The model under review builds one solid part; all positions refer to its coordinate system, in mm. Round coordinates to 2 decimals unless told otherwise and drop trailing zeros. Loops run counter-clockwise (first coordinate to the right, second up) from the corner with the lowest first, then second, coordinate; pieces in that order, holes last. Notation, with made-up numbers: (50.25, 79.5) -> (55.25, 79.5) arc R15 cw to (55.25, 96.5) -> close; hole circle Ø2 at (79, 71). An arc over 180 degrees is marked (long way). Use a Markdown table: item, result. Add a question column.
1) Wall thickness on probe 1 along Z at (x, y) = (23, 8); probe 2 along Y at (x, z) = (-73, -15); probe 3 along Z at (x, y) = (-37, -3.5): over which ranges is each line inside the solid? List them lowest first.
2) Insertion check: pin 1 (3.5 mm diameter, centred on x = 23.32, z = 0.42, fed in from +Y) (3 decimals). The pin has a flat end and moves straight along its axis. Give the tip position at first contact, or say it passes through.
3) Consider section B-B on z = 17.5. Give the boundary of the cut face in (x, y), plus the area to 3 significant figures.
4) Consider section A-A on y = -1.5. Give the boundary of the cut face in (x, z), plus the area to 3 significant figures.
5) Consider section C-C on x = -86.5. Give the boundary of the cut face in (y, z), plus the area to 3 significant figures.
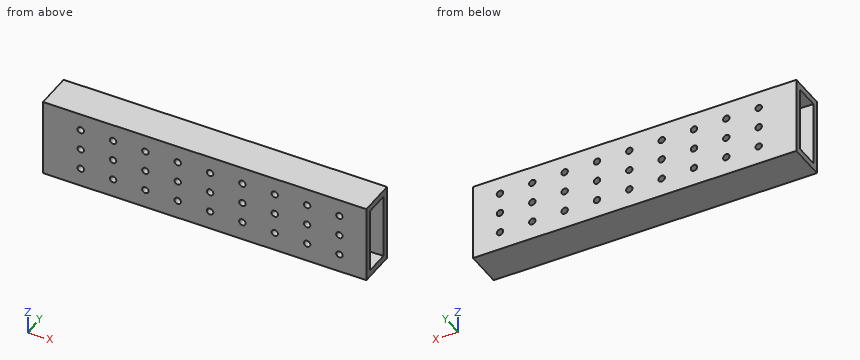
from build123d import *

# Parameters (mm, degrees)
SKETCH1_W           = 48
SKETCH1_H           = 23
SKETCH1_W_2         = 40
SKETCH1_H_2         = 15
EXTRUDE_THIN1_DEPTH = 100
SKETCH2_R           = 2
CUT_EXTRUDE1_DEPTH  = 24


with BuildPart() as part:
    # Sketch1 → Extrude-Thin1 (new body, symmetric)
    with BuildSketch(Plane(origin=(0, 0, 0), x_dir=(0, 0, -1), z_dir=(1, 0, 0))):
        Rectangle(SKETCH1_W, SKETCH1_H)
        Rectangle(SKETCH1_W_2, SKETCH1_H_2, mode=Mode.SUBTRACT)
    extrude(amount=EXTRUDE_THIN1_DEPTH, both=True)

    # Sketch2 → Cut-Extrude1 (cut, through all)
    with BuildSketch(Plane(origin=(0, 11.5, 0), x_dir=(1, 0, 0), z_dir=(0, 1, 0))):
        with Locations((-76.678469137, 12.583133397)):
            Circle(SKETCH2_R)
        with Locations((-56.678469137, 12.583133397)):
            Circle(SKETCH2_R)
        with Locations((-36.678469137, 12.583133397)):
            Circle(SKETCH2_R)
        with Locations((-16.678469137, 12.583133397)):
            Circle(SKETCH2_R)
        with Locations((3.321530863, 12.583133397)):
            Circle(SKETCH2_R)
        with Locations((23.321530863, 12.583133397)):
            Circle(SKETCH2_R)
        with Locations((43.321530863, 12.583133397)):
            Circle(SKETCH2_R)
        with Locations((63.321530863, 12.583133397)):
            Circle(SKETCH2_R)
        with Locations((83.321530863, 12.583133397)):
            Circle(SKETCH2_R)
        with Locations((-56.678469137, -0.416866603)):
            Circle(SKETCH2_R)
        with Locations((-36.678469137, -0.416866603)):
            Circle(SKETCH2_R)
        with Locations((-16.678469137, -0.416866603)):
            Circle(SKETCH2_R)
        with Locations((3.321530863, -0.416866603)):
            Circle(SKETCH2_R)
        with Locations((23.321530863, -0.416866603)):
            Circle(SKETCH2_R)
        with Locations((43.321530863, -0.416866603)):
            Circle(SKETCH2_R)
        with Locations((63.321530863, -0.416866603)):
            Circle(SKETCH2_R)
        with Locations((83.321530863, -0.416866603)):
            Circle(SKETCH2_R)
        with Locations((-56.678469137, -13.416866603)):
            Circle(SKETCH2_R)
        with Locations((-36.678469137, -13.416866603)):
            Circle(SKETCH2_R)
        with Locations((-16.678469137, -13.416866603)):
            Circle(SKETCH2_R)
        with Locations((3.321530863, -13.416866603)):
            Circle(SKETCH2_R)
        with Locations((23.321530863, -13.416866603)):
            Circle(SKETCH2_R)
        with Locations((43.321530863, -13.416866603)):
            Circle(SKETCH2_R)
        with Locations((63.321530863, -13.416866603)):
            Circle(SKETCH2_R)
        with Locations((83.321530863, -13.416866603)):
            Circle(SKETCH2_R)
        with Locations((-76.678469137, -0.416866603)):
            Circle(SKETCH2_R)
        with Locations((-76.678469137, -13.416866603)):
            Circle(SKETCH2_R)
    extrude(amount=-CUT_EXTRUDE1_DEPTH, mode=Mode.SUBTRACT)


solid = part.part
Result set:
| question | item | result |
|---|---|---|
| 1 | probe 1 | -24 to -14.56, -10.61 to -1.56, 2.39 to 11.44, 15.39 to 24 |
| 1 | probe 2 | -11.5 to -7.5, 7.5 to 11.5 |
| 1 | probe 3 | -24 to -20, 20 to 24 |
| 2 | pin 1 | through |
| 3 | outline | (-100, -11.5) -> (100, -11.5) -> (100, -7.5) -> (-100, -7.5) -> close; (-100, 7.5) -> (100, 7.5) -> (100, 11.5) -> (-100, 11.5) -> close |
| 3 | area | 1,600 mm2 |
| 4 | outline | (-100, -24) -> (100, -24) -> (100, -20) -> (-100, -20) -> close; (-100, 20) -> (100, 20) -> (100, 24) -> (-100, 24) -> close |
| 4 | area | 1,600 mm2 |
| 5 | outline | (-11.5, -24) -> (11.5, -24) -> (11.5, 24) -> (-11.5, 24) -> close; hole (-7.5, -20) -> (7.5, -20) -> (7.5, 20) -> (-7.5, 20) -> close |
| 5 | area | 504 mm2 |
